```python
from build123d import *

# Parameters (mm, degrees)
SKETCH1_W           = 154
SKETCH1_H           = 56
PLATE_DEPTH         = 10
BOSS_EXTRUDE1_DEPTH = 20
CORNER_START        = -15
CORNER_DEPTH        = 5
CORNER2_START       = 15
CORNER2_DEPTH       = 5
SKETCH3_R           = 4
CUT_EXTRUDE1_DEPTH  = 28
FILLET1_R           = 5


with BuildPart() as part:
    # Sketch1 → plate (new body)
    with BuildSketch(Plane(origin=(0, 0, 0), x_dir=(1, 0, 0), z_dir=(0, 1, 0))):
        Rectangle(SKETCH1_W, SKETCH1_H)
    extrude(amount=PLATE_DEPTH)

    # Sketch2 → Boss-Extrude1 (add, symmetric)
    with BuildSketch(Plane.XY):
        Polygon((-8, 10), (-8, 38), (-14, 38), (-14, 16), (-36, 16), (-36, 10), align=None)
        Polygon((36, 16), (36, 10), (8, 10), (8, 38), (14, 38), (14, 16), align=None)
    extrude(amount=BOSS_EXTRUDE1_DEPTH, both=True)

    # Sketch2<4> → Corner (add)
    with BuildSketch(Plane.XY.offset(CORNER_START)):
        Polygon((-14, 16), (-14, 31), (-29, 16), align=None)
        Polygon((29, 16), (14, 31), (14, 16), align=None)
    extrude(amount=-CORNER_DEPTH)

    # Sketch2<3> → Corner2 (add)
    with BuildSketch(Plane.XY.offset(CORNER2_START)):
        Polygon((-14, 16), (-14, 31), (-29, 16), align=None)
        Polygon((29, 16), (14, 31), (14, 16), align=None)
    extrude(amount=CORNER2_DEPTH)

    # Sketch3 → Cut-Extrude1 (cut)
    with BuildSketch(Plane.ZY.offset(14)):
        with Locations((0, 28)):
            Circle(SKETCH3_R)
    extrude(amount=-CUT_EXTRUDE1_DEPTH, mode=Mode.SUBTRACT)

    # Fillet1
    fillet1_edges = [part.edges().sort_by_distance(p)[0] for p in [
        (-11, 38, -20),
        (-11, 38, 20),
        (11, 38, 20),
        (11, 38, -20),
    ]]
    fillet(fillet1_edges, radius=FILLET1_R)


solid = part.part
```
Can you work these out from the model? Positions are in its coordinate system, mm. A direction names the side the tool comes from. Give positions to 0.01 mm unless a question says otherwise; leave off trailing zeros. Write each loop counter-clockwise with the first axis right and the second up, starting at its lowest first coordinate (ties: lowest second). Pieces come first, ordered by that corner, then holes. Notation, with made-up numbers: (47.5, 9) -> (99.5, 9) arc R13 ccw to (99.5, 28) -> close; hole circle Ø5 at (2, -12.5). An arc over 180 degrees is marked (long way). One line per item, written item: value.
Q1. Imagine slicing it at D-D on x = 15.5. Please give me the cut outline in (y, z).
Results found:
outline: (0, -28) -> (10, -28) -> (10, -20) -> (29.5, -20) -> (29.5, -15) -> (16, -15) -> (16, 15) -> (29.5, 15) -> (29.5, 20) -> (10, 20) -> (10, 28) -> (0, 28) -> close
Q2. Imagine slicing it at C-C on z = 0. Please give me the cut outline in (x, y), and give its area (3 significant figures).
Results found:
outline: (-77, 0) -> (77, 0) -> (77, 10) -> (36, 10) -> (36, 16) -> (14, 16) -> (14, 24) -> (8, 24) -> (8, 10) -> (-8, 10) -> (-8, 24) -> (-14, 24) -> (-14, 16) -> (-36, 16) -> (-36, 10) -> (-77, 10) -> close; (-14, 32) -> (-8, 32) -> (-8, 38) -> (-14, 38) -> close; (8, 32) -> (14, 32) -> (14, 38) -> (8, 38) -> close
area: 2,040 mm^2
Q3. Which directions (+Z, -Z, +X, -X, +Y, -Y) give clear straight access to the entire face, cutting with the end or side of a thin tool? Please do faces 4 (the face through (-18, 20, 15)), 5 (the face through (19, 19, 20)), 6 (the face through (-8, 23.8, -0.3)), 7 (the face through (14, 27.2, -4.2)).
Results found:
face 4: -X, +Y
face 5: +Z, +X, -X, +Y
face 6: +Z, -Z, +Y
face 7: +X, +Y
Q4. Please list where these lines run through material, in increasing order: line 1 (Y direction, x = -11.35, z = 0); line 2 (X direction, y = 32, z = 16); line 3 (Y direction, x = 46, z = -24.5). Write a range as [from, to].
Results found:
line 1: y = [0, 24], [32, 38]
line 2: x = [-14, -8], [8, 14]
line 3: y = [0, 10]
Q5. We'd pull the mould along Z, two halves only. Please class faces 1 (the face through (-19, 19, 20)), 2 (the face through (-25, 16, 0)), 3 (the face through (-77, 5, 0)): +Z half, -Z half, draft (parallel to the pull), parting line (faces both ways), or undercut.
Results found:
face 1: +Z half
face 2: undercut
face 3: draft
Q6. Imagine slicing it at B-B on y = 28. Please give me the cut outline in (x, z).
Results found:
outline: (-17, -20) -> (-8, -20) -> (-8, -4) -> (-14, -4) -> (-14, -15) -> (-17, -15) -> close; (-17, 15) -> (-14, 15) -> (-14, 4) -> (-8, 4) -> (-8, 20) -> (-17, 20) -> close; (8, -20) -> (17, -20) -> (17, -15) -> (14, -15) -> (14, -4) -> (8, -4) -> close; (8, 4) -> (14, 4) -> (14, 15) -> (17, 15) -> (17, 20) -> (8, 20) -> close
Q7. Imagine slicing it at A-A on y = 17.5. Please give me the cut outline in (x, z).
Results found:
outline: (-27.5, -20) -> (-8, -20) -> (-8, 20) -> (-27.5, 20) -> (-27.5, 15) -> (-14, 15) -> (-14, -15) -> (-27.5, -15) -> close; (8, -20) -> (27.5, -20) -> (27.5, -15) -> (14, -15) -> (14, 15) -> (27.5, 15) -> (27.5, 20) -> (8, 20) -> close
Q8. For P1, Ø7, axis at x = -24, y = 22, coming from the -Z side; P2, Ø1, axis at y = 18.5, z = -17.5, coming from the +X side; P3, Ø7, axis at y = 28, z = 0, coming from the +X side; P4, Ø3, axis at y = 14, z = -4, coming from the +X side, each with a flat end and sliding along its axis, tell me the tip position at first contact or that it passes through.
Results found:
P1: stops at z = -20
P2: stops at x = 27
P3: passes through
P4: stops at x = 36
